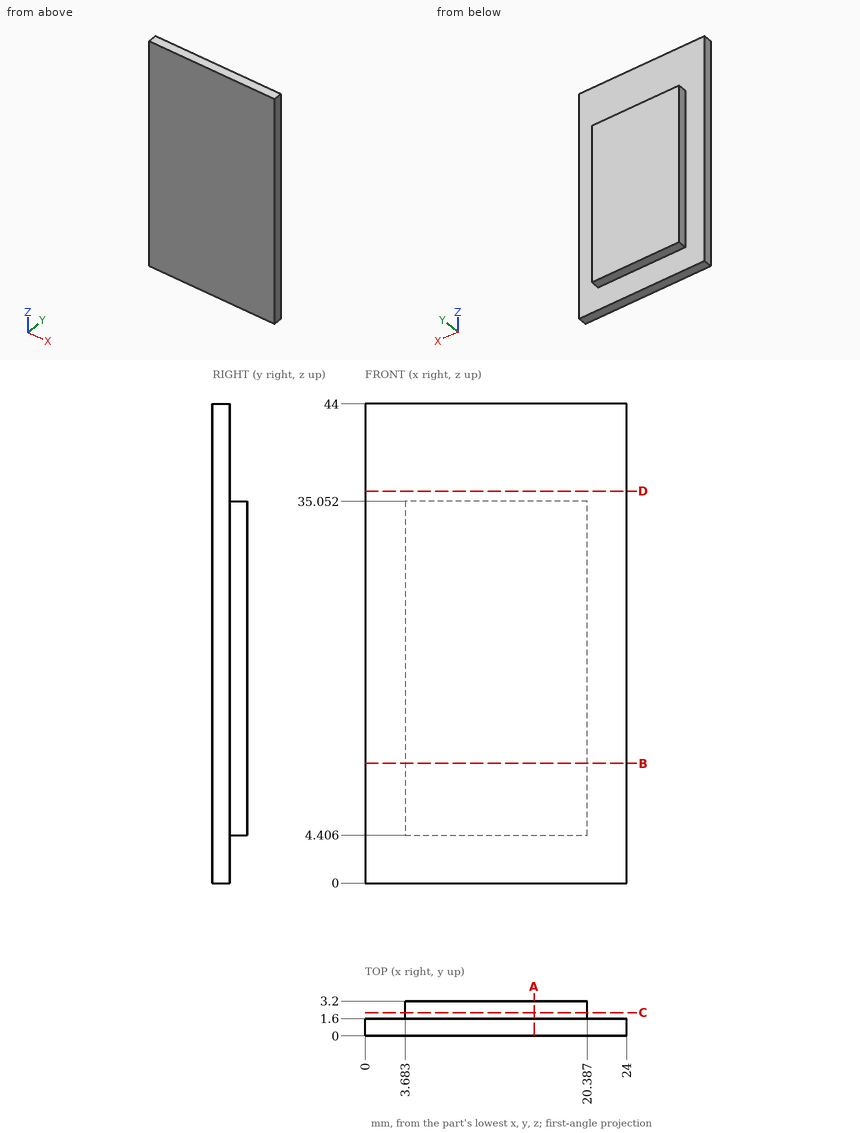
The figure shows three views and two pictorial views of one solid part (mm, origin at its lowest corner). Answer the questions. Give positions to 0.01 mm unless a question says otherwise; leave off trailing zeros. Loops run counter-clockwise (first coordinate to the right, second up) from the corner with the lowest first, then second, coordinate; pieces in that order, holes last. Notation, with made-up numbers: (49, 85.25) -> (54, 85.25) arc R10 ccw to (54, 98.25) -> close; hole circle Ø1 at (22.5, 75). An arc over 180 degrees is marked (long way). Use a Markdown table: item, result. Add a question column.
1. Section D-D on z = 36 is taken. Determine the outline of the cut face in (x, y), and give its area (3 significant figures).
2. Flat-ended cylindrical pins translate along their axes: pin 1 Ø0.8 at (y, z) = (3, 22) entering from -X; pin 2 Ø0.5 at (x, y) = (8.5, 2) entering from +Z; pin 3 Ø1.5 at (y, z) = (2.5, 11) entering from +X. Find the tip coordinate at first contact, or state that the pin passes through.
3. Section A-A on x = 15.5 is taken. Determine the outline of the cut face in (y, z), and give its area (3 significant figures).
4. Find the intervals of material crossed by probe 1 along Z at (x, y) = (18, 1.75); probe 2 along X at (y, z) = (1.8, 19); probe 3 along Y at (x, z) = (11, 36), in increasing order.
5. Section C-C on y = 2.15 is taken. Determine the outline of the cut face in (x, z).
6. Section B-B on z = 11 is taken. Determine the outline of the cut face in (x, y).
Results below:
| question | item | result |
|---|---|---|
| 1 | outline | (0, 0) -> (24, 0) -> (24, 1.6) -> (0, 1.6) -> close |
| 1 | area | 38.4 mm^2 |
| 2 | pin 1 | stops at x = 3.68 |
| 2 | pin 2 | stops at z = 35.05 |
| 2 | pin 3 | stops at x = 20.39 |
| 3 | outline | (0, 0) -> (1.6, 0) -> (1.6, 4.41) -> (3.2, 4.41) -> (3.2, 35.05) -> (1.6, 35.05) -> (1.6, 44) -> (0, 44) -> close |
| 3 | area | 119 mm^2 |
| 4 | probe 1 | z = 4.41 to 35.05 |
| 4 | probe 2 | x = 3.68 to 20.39 |
| 4 | probe 3 | y = 0 to 1.6 |
| 5 | outline | (3.68, 4.41) -> (20.39, 4.41) -> (20.39, 35.05) -> (3.68, 35.05) -> close |
| 6 | outline | (0, 0) -> (24, 0) -> (24, 1.6) -> (20.39, 1.6) -> (20.39, 3.2) -> (3.68, 3.2) -> (3.68, 1.6) -> (0, 1.6) -> close |
